from build123d import *

# Parameters (mm, degrees)
SKETCH1_W           = 75
SKETCH1_H           = 75
SKETCH1_R           = 5.5
SKETCH1_R_2         = 20
BOSS_EXTRUDE1_DEPTH = 6


with BuildPart() as part:
    # Sketch1 → Boss-Extrude1 (new body)
    with BuildSketch(Plane(origin=(0, 0, 0), x_dir=(0, 0, -1), z_dir=(1, 0, 0))):
        Rectangle(SKETCH1_W, SKETCH1_H)
        with Locations((25, 25)):
            Circle(SKETCH1_R, mode=Mode.SUBTRACT)
        with Locations(Location((-25, 25, 0), (0, 0, 180))):
            Circle(SKETCH1_R, mode=Mode.SUBTRACT)
        with Locations(Location((25, -25, 0), (0, 0, 180))):
            Circle(SKETCH1_R, mode=Mode.SUBTRACT)
        with Locations((-25, -25)):
            Circle(SKETCH1_R, mode=Mode.SUBTRACT)
        Circle(SKETCH1_R_2, mode=Mode.SUBTRACT)
    extrude(amount=BOSS_EXTRUDE1_DEPTH)


solid = part.part
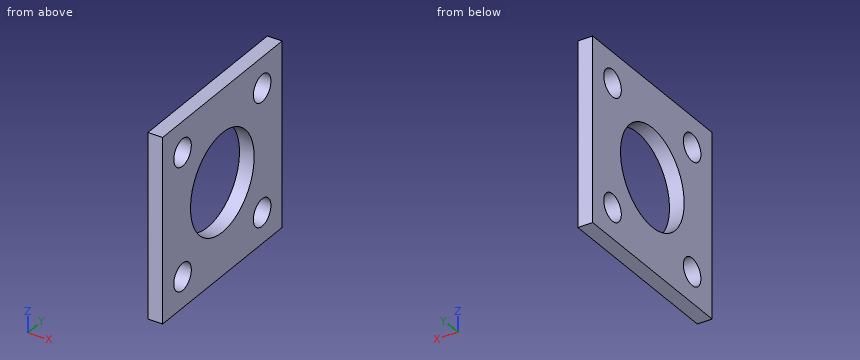
Design review of the part built by this model. Coordinates are the model's own, in mm. Coordinates: 2 decimals unless noted, no trailing zeros. Loops run counter-clockwise (first coordinate to the right, second up) from the corner with the lowest first, then second, coordinate; pieces in that order, holes last. Notation, with made-up numbers: M 6.25,63 L 56.25,63 A14 cw 56.25,83 Z; hole C 19,31 d1. An arc over 180 degrees is marked long. Answer as CSV lines item,"result".
Item 1: Add section D-D on x = 1.35. State the section outline as (y, z) points.
Answer list:
outline,"M -37.5,-37.5 L 37.5,-37.5 L 37.5,37.5 L -37.5,37.5 Z; hole C -25,-25 d11; hole C -25,25 d11; hole C 0,0 d40; hole C 25,-25 d11; hole C 25,25 d11"
Item 2: Add section A-A on z = -25. State the section outline as (x, y) points.
Answer list:
outline,"M 0,-37.5 L 6,-37.5 L 6,-30.5 L 0,-30.5 Z; M 0,-19.5 L 6,-19.5 L 6,19.5 L 0,19.5 Z; M 0,30.5 L 6,30.5 L 6,37.5 L 0,37.5 Z"
Item 3: Add section B-B on z = 0. State the section outline as (x, y) points, plus the area to 3 significant figures.
Answer list:
outline,"M 0,-37.5 L 6,-37.5 L 6,-20 L 0,-20 Z; M 0,20 L 6,20 L 6,37.5 L 0,37.5 Z"
area,"210 mm²"
Item 4: For probe 1 along Y at (x, z) = (3, -25); probe 2 along Y at (x, z) = (2.45, -22.5); probe 3 along Y at (x, z) = (4.25, -4), list the stretches that pass through material, from the lowest coordinate up.
Answer list:
probe 1,"-37.5 to -30.5, -19.5 to 19.5, 30.5 to 37.5"
probe 2,"-37.5 to -29.9, -20.1 to 20.1, 29.9 to 37.5"
probe 3,"-37.5 to -19.6, 19.6 to 37.5"
